Input: part model. Units: mm. Frame: model coordinates. Face numbers are marked on the shaded views. A direction names the side the tool comes from. Coordinates: 2 decimals unless noted, no trailing zeros. Order: outer loops, then holes, each group sorted by start corner. A loop starts at its lowest first (then second) coordinate and runs counter-clockwise, first axis right, second up. Notation, with made-up numbers: (36, -27) - (40, -27) arc R12 cw to (40, -8) - close; hole circle Ø4 at (88, 9.25). An arc over 180 degrees is marked (long way). Use a Markdown table: item, result. Add a question column.
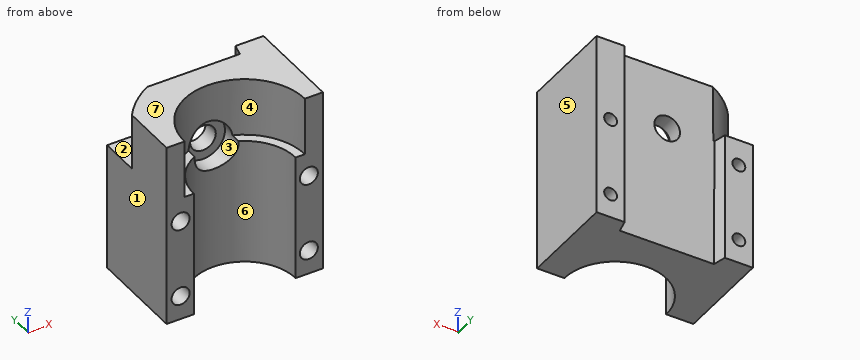
Autodesk Inventor part; units mm, degrees
ref_plane "YZ Plane" through (0, 0, 0) normal (1, 0, 0) x (0, 1, 0)
ref_plane "XZ Plane" through (0, 0, 0) normal (0, 1, 0) x (-1, 0, 0)
ref_plane "XY Plane" through (0, 0, 0) normal (0, 0, 1) x (1, 0, 0)
sketch "スケッチ1" plane through (0, 0, 0) normal (0, 0, 1) x (1, 0, 0)
  line L0 (-12.5, 3.2) -> (-11.75, 0)
  line L1 (-11.75, 0) -> (11.75, 0)
  line L2 (11.75, 0) -> (12.5, 3.2)
  line L3 (12.5, 3.2) -> (19.5, 3.2)
  line L4 (19.5, 3.2) -> (19.5, -4)
  line L5 (19.5, -4) -> (-19.5, -4)
  line L6 (-19.5, -4) -> (-19.5, 3.2)
  line L7 (-19.5, 3.2) -> (-12.5, 3.2)
  circle A0 centre (0, -21) radius 12.7 construction
  line L8 (-5.5, -4) -> (5.5, -4) construction
  line L9 (5.5, -4) -> (5.5, -7.5) construction
  line L10 (5.5, -7.5) -> (-5.5, -7.5) construction
  line L11 (-5.5, -7.5) -> (-5.5, -4) construction
  circle A1 centre (0, -21) radius 14.7 construction
  line L12 (-19.5, -21) -> (19.5, -21) construction
  line L13 (-18.75, -24.8) -> (-13.25, -24.8) construction
  line L14 (-13.25, -24.8) -> (-13.25, -27.8) construction
  line L15 (-13.25, -27.8) -> (-18.75, -27.8) construction
  line L16 (-18.75, -27.8) -> (-18.75, -24.8) construction
  line L17 (-16, -27.8) -> (-16, -14.8) construction
  line L18 (-18.75, -14.8) -> (-13.25, -14.8) construction
  line L19 (-13.25, -14.8) -> (-13.25, -17.2) construction
  line L20 (-13.25, -17.2) -> (-18.75, -17.2) construction
  line L21 (-18.75, -17.2) -> (-18.75, -14.8) construction
  line L22 (-14.5, -14.8) -> (-14.5, -27.8) construction
  line L23 (-17.5, -14.8) -> (-17.5, -27.8) construction
  point P0 (0, 0)
  point P1 (0, 0)
  point P2 (0, -4)
  dimension "d0" = 4
  dimension "d1" = 3.2
  dimension "d2" = 23.5
  dimension "d3" = 25
  dimension "d4" = 39
  dimension "d5" = 25.4
  dimension "d6" = 3.5
  dimension "d7" = 21
  dimension "d8" = 11
  dimension "d9" = 2
  dimension "d11" = 5.5
  dimension "d12" = 3
  dimension "d13" = 5.5
  dimension "d14" = 2.4
  dimension "d15" = 10
  dimension "d16" = 1.5
  dimension "d17" = 1.5
  dimension "d18" = 3.8
  dimension "d19" = 16
extrude "押し出し1" add sketch "スケッチ1" along normal blind 46
sketch "スケッチ2" plane through (0, 0, 0) normal (0, 0, -1) x (-1, 0, 0)
  line L0 (19.5, -4) -> (-19.5, -4)
  circle A0 centre (0, -21) radius 12.7
  line L1 (19.5, -21) -> (-19.5, -21)
  line L2 (-19.5, -21) -> (-19.5, -4)
  line L3 (19.5, -4) -> (19.5, -21)
  point P0 (0, 0)
  point P1 (-12.7, -21)
  point P2 (12.7, -21)
extrude "押し出し2" add sketch "スケッチ2" against normal blind 31.5 contours L3 L1 A0 L2 L0
sketch "スケッチ3" plane through (0, 0, 31.5) normal (0, 0, 1) x (1, 0, 0)
  line L0 (-19.5, -4) -> (19.5, -4)
  line L1 (-19.5, -4) -> (-19.5, -21)
  line L2 (-19.5, -21) -> (-12.7, -21)
  arc A0 (12.7, -21) -> (-12.7, -21) centre (0, -21) ccw
  line L3 (12.7, -21) -> (19.5, -21)
  line L4 (19.5, -21) -> (19.5, -4)
  circle A1 centre (0, -21) radius 15
  point P0 (0, 0)
  point P1 (-15, -21)
  point P2 (15, -21)
  dimension "d24" = 30
extrude "押し出し3" add sketch "スケッチ3" along normal up to surface (14.5 mm away) contours L0 L4 L3 A1 L2 L1
sketch "スケッチ5" plane through (0, 0, 0) normal (0, 1, 0) x (-1, 0, 0)
  circle A0 centre (0, 31) radius 5.5
  line L0 (-11.75, 46) -> (11.75, 46)
  point P0 (0, 0)
  point P1 (0, 46)
  dimension "d27" = 15
  dimension "d28" = 11
extrude "押し出し4" cut sketch "スケッチ5" along normal through all both and the other way through all
sketch "スケッチ6" plane through (-11.75, 0, 0) normal (0, 1, 0) x (1, 0, 0)
  circle A0 centre (11.75, -31) radius 5.5
  circle A1 centre (11.75, -31) radius 3.2
  point P0 (11.75, 0)
  dimension "d31" = 6.4
extrude "押し出し5" add sketch "スケッチ6" against normal blind 4
sketch "スケッチ7" plane through (-19.5, -21, 0) normal (0, -1, 0) x (1, 0, 0)
  line L0 (6.8, 0) -> (0, 0) construction
  line L1 (6.8, 0) -> (6.8, 31.5) construction
  line L2 (4.5, 31.5) -> (6.8, 31.5) construction
  line L3 (4.5, 31.5) -> (4.5, 46) construction
  line L4 (4.5, 46) -> (0, 46) construction
  line L5 (0, 0) -> (0, 46) construction
  line L6 (3.5, 0) -> (3.5, 31.5) construction
  circle A0 centre (3.5, 6) radius 2.25
  circle A1 centre (3.5, 25.5) radius 2.25
  point P0 (19.5, 0)
  dimension "d34" = 16
  dimension "d35" = 4.5
  dimension "d36" = 6
  dimension "d37" = 6
extrude "押し出し6" cut sketch "スケッチ7" against normal blind 5
sketch "スケッチ8" plane through (-16, -16, 6) normal (0, -1, 0) x (1, 0, 0)
  circle A0 centre (0, 0) radius 2.25
  circle A1 centre (0, 19.5) radius 2.25
  circle A2 centre (0, 0) radius 1.6
  circle A3 centre (0, 19.5) radius 1.6
  point P0 (16, -6)
  dimension "d40" = 3.2
extrude "押し出し7" cut sketch "スケッチ8" against normal through all contours A2 | A3
mirror "ミラー1" about plane through (0, 0, 0) normal (1, 0, 0) of "押し出し7", "押し出し6"
sketch "スケッチ9" plane through (-11.75, 0, 0) normal (0, 1, 0) x (1, 0, 0)
  line L0 (-7.75, -46) -> (3.9203, -46)
  line L1 (3.9203, -46) -> (3.9203, -32)
  line L2 (3.9203, -32) -> (-7.75, -32)
  line L3 (-7.75, -32) -> (-7.75, -46)
  point P0 (11.75, 0)
  dimension "d43" = 14
extrude "押し出し8" cut sketch "スケッチ9" along normal blind 10
sketch "スケッチ10" plane through (0, 0, 0) normal (1, 0, 0) x (0, 1, 0)
  line L0 (0, 0) -> (0, 46)
  line L1 (3.2, 46) -> (-21, 46)
  line L2 (3.2, 0) -> (-21, 0)
  line L3 (0, 0) -> (0.2, 46)
  dimension "d46" = 0.2
extrude "押し出し9" add sketch "スケッチ10" along normal up to surface surface through (12.5, 3.2, 0) normal (-0.9736163, 0.2281913, 0)
mirror "ミラー2" about plane through (0, 0, 0) normal (1, 0, 0) of "押し出し9"
sketch "スケッチ11" plane through (0, -4, 31) normal (0, -1, 0) x (1, 0, 0)
  circle A0 centre (0, 0) radius 3.2
  point P0 (0, -31)
extrude "押し出し10" cut sketch "スケッチ11" against normal through all
sketch "スケッチ12" plane through (0, 0, 46) normal (0, 0, 1) x (1, 0, 0)
  arc A0 (15, -21) -> (-15, -21) centre (0, -21) ccw
  arc A1 (-11.3852, 0.2) -> (-19.5, -6.8999) centre (0, -21) ccw
  line L0 (-19.5, 0) -> (-19.5, -21)
  line L1 (-19.5, 0) -> (-19.5, 3.2)
  line L2 (-19.5, 3.2) -> (-12.5, 3.2)
  line L3 (-12.5, 3.2) -> (-11.7826, 0.1391)
  line L4 (11.7969, 0.2) -> (-11.7969, 0.2)
  point P0 (0, 0)
  point P1 (-11.75, 0)
extrude "押し出し11" cut sketch "スケッチ12" against normal up to surface (14 mm away)
equation "\"d17\" = d16"
equation "\"d32\" = d0"
properties part number "led_holder_01"
1) Cut plane A-A (x = 16). Return the cut outline in (y, z), and give its area (3 significant figures).
2) Cut plane D-D (z = 33). Return the cut outline in (x, y).
3) Contact query for flat-ended pins moving along their axis: P1, Ø2, axis at x = 15, z = 26, coming from the -Y side; P2, Ø3, axis at x = -2, z = 5, coming from the -Y side; P3, Ø14.5, axis at x = 0, z = 31, coming from the +Y side. Output: stop coordinate, or through.
4) Cut plane B-B (y = -12). Return the cut outline in (x, z).
5) Material intervals for L1, parallel to Z at x = -16, y = -2.25; L2, parallel to Z at x = -15, y = -17; L3, parallel to X at y = -6.8, z = 31, sorted ascending.
6) Cut plane C-C (z = 6). Return the cut outline in (x, y), and give its area (3 significant figures).
7) Pull-direction query (X, two-part tool) for the marked faces 4, 5, 6 and 7; classes: pulls with the +X half, pulls with the -X half, needs draft (parallel to the pull), parting line crosses it, or undercut.
8) Reachability of the marked faces 1, 2 and 3 from +Z, -Z, +X, -X, +Y, -Y: full face, straight path, thin tool, end or side. Return the list, or none.
Computed:
| question | item | result |
|---|---|---|
| 1 | outline | (-21, 0) - (3.2, 0) - (3.2, 4.4) - (-16, 4.4) - (-16, 3.75) - (-21, 3.75) - close; (-21, 8.25) - (-16, 8.25) - (-16, 7.6) - (3.2, 7.6) - (3.2, 23.9) - (-16, 23.9) - (-16, 23.25) - (-21, 23.25) - close; (-21, 27.75) - (-16, 27.75) - (-16, 27.1) - (3.2, 27.1) - (3.2, 46) - (-21, 46) - close |
| 1 | area | 945 mm2 |
| 2 | outline | (-19.5, -21) - (-15, -21) arc R15 cw to (-5.12, -6.9) - (-5.12, -4) - (-2.5, -4) - (-2.5, 0.14) - (-11.49, 0.14) arc R24.06 ccw to (-19.5, -6.9) - close; (2.5, -4) - (5.12, -4) - (5.12, -6.9) arc R15 cw to (15, -21) - (19.5, -21) - (19.5, 3.2) - (12.5, 3.2) - (11.78, 0.14) - (2.5, 0.14) - close |
| 3 | P1 | stops at y = -16 |
| 3 | P2 | stops at y = -8.79 |
| 3 | P3 | stops at y = 0.17 |
| 4 | outline | (-19.5, 0) - (-8.96, 0) - (-8.96, 31.5) - (-12, 31.5) - (-12, 46) - (-19.5, 46) - close; (8.96, 0) - (19.5, 0) - (19.5, 46) - (12, 46) - (12, 31.5) - (8.96, 31.5) - close; hole circle Ø3.2 at (-16, 6); hole circle Ø3.2 at (-16, 25.5); hole circle Ø3.2 at (16, 6); hole circle Ø3.2 at (16, 25.5) |
| 5 | L1 | z = 0 to 4.4, 7.6 to 23.9, 27.1 to 32 |
| 5 | L2 | z = 0 to 3.98, 8.02 to 23.48, 27.52 to 46 |
| 5 | L3 | x = -19.5 to -5.5, 5.5 to 19.5 |
| 6 | outline | (-19.5, -21) - (-18.25, -21) - (-18.25, -16) - (-17.6, -16) - (-17.6, 3.2) - (-19.5, 3.2) - close; (-14.4, -16) - (-13.75, -16) - (-13.75, -21) - (-12.7, -21) arc R12.7 cw to (12.7, -21) - (13.75, -21) - (13.75, -16) - (14.4, -16) - (14.4, 3.2) - (12.5, 3.2) - (11.76, 0.03) - (-11.76, 0.03) - (-12.5, 3.2) - (-14.4, 3.2) - close; (17.6, -16) - (18.25, -16) - (18.25, -21) - (19.5, -21) - (19.5, 3.2) - (17.6, 3.2) - close |
| 6 | area | 446 mm2 |
| 7 | face 4 | undercut |
| 7 | face 5 | pulls with the +X half |
| 7 | face 6 | undercut |
| 7 | face 7 | needs draft |
| 8 | face 1 | +Z, -Z, -X, +Y, -Y |
| 8 | face 2 | +Z, -X, +Y |
| 8 | face 3 | -Y |
